Part model, mm, in its own coordinate system. Face numbers are marked on the shaded views. A direction names the side the tool comes from. Round coordinates to 2 decimals unless told otherwise and drop trailing zeros. Order: outer loops, then holes, each group sorted by start corner. A loop starts at its lowest first (then second) coordinate and runs counter-clockwise, first axis right, second up. Notation, with made-up numbers: (14, 21) -> (29, 21) arc R5 cw to (29, 30) -> close; hole circle Ø11 at (75, 31). An arc over 180 degrees is marked (long way). Use CSV: the item, a comma, the result in double quotes.
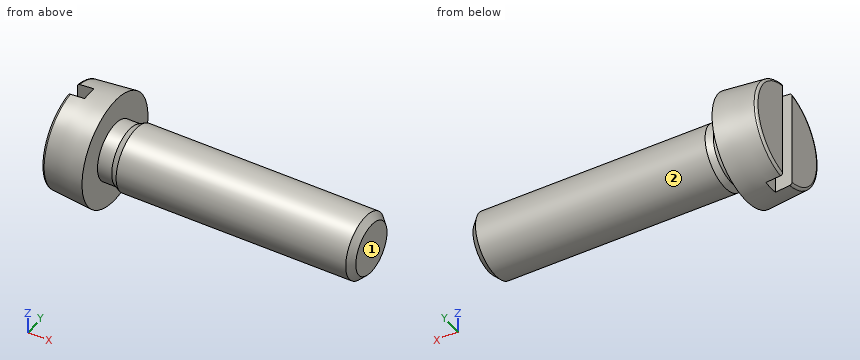
Autodesk Inventor part; units mm, degrees
ref_plane "Work Plane1" through (30.1625, 0, 0) normal (0, 0, -1) x (1, 0, 0)
ref_plane "YZ Plane" through (0, 0, 0) normal (1, 0, 0) x (0, 1, 0)
ref_plane "XZ Plane" through (0, 0, 0) normal (0, 1, 0) x (-1, 0, 0)
sketch "Sketch1" plane through (0, 0, 0) normal (0, 0, 1) x (1, 0, 0)
  line L0 (-3.3, 0) -> (20, 0)
  line L1 (20, 0) -> (20, 2.5)
  line L2 (20, 2.5) -> (1.6, 2.5)
  line L3 (1.6, 2.5) -> (1.1091, 2.2547)
  line L4 (1.1091, 2.2547) -> (0, 2.2547)
  line L5 (0, 2.2547) -> (0, 4.25)
  line L6 (-7.96, 0) -> (24.66, 0)
  line L7 (0, -0.85) -> (0, 5.1)
  line L8 (-3.3, 0) -> (-3.3, 3.9613)
  line L9 (0, 4.25) -> (-3.3, 3.9613)
  line L10 (1.6, 2.5) -> (0, 2.5) construction
  dimension "d0" = 20
  dimension "d1" = 18.4
  dimension "d2" = 0.4909
  dimension "d3" = 3.3
  dimension "d4" = 5
  dimension "d5" = 4.5095
  dimension "d9" = 8.5
  dimension "d10" = 5
revolve "Body" add sketch "Sketch1" angle 360 about axis through (-3.3, 0, 0) along (1, 0, 0)
sketch "Sketch2" plane through (-3.3, 0, 0) normal (-1, 0, 0) x (0, 0, 1)
  circle A0 centre (0, 0) radius 4.25
  line L0 (0, 0) -> (0, 3.9613)
  line L1 (-4.25, 0.6) -> (4.25, 0.6)
  line L2 (4.25, 0.6) -> (4.25, -0.6)
  line L3 (4.25, -0.6) -> (-4.25, -0.6)
  line L4 (-4.25, -0.6) -> (-4.25, 0.6)
  line L5 (-4.25, 0) -> (4.25, 0) construction
  line L6 (0, 0.6) -> (0, -0.6) construction
  point P0 (0, 0)
  dimension "d11" = 1.2
  dimension "d12" = 8.5
fillet "Fillet1" radius 0.2 1 edges at (-3.3, -3.9613, 0)
extrude "Slot" cut sketch "Sketch2" against normal blind 1.3 contours A0 L3 L1 | L2 L3 A0 | A0 L1 L2 | A0 L4 L1 | L3 L4 A0
thread "Thread"
chamfer "Chamfer1" distance 0.4908 distance2 0.4909 1 edges at (20, -2.5, 0) measured on face at (20, 1.2612, -0.6619)
ref_plane "Work Plane1" through (30.1625, 0, 0) normal (0, 0, -1) x (1, 0, 0)
equation "\"d11\" = SBR"
equation "\"d12\" = KOD"
equation "\"d19\" = STI"
equation "\"d14\" = RR"
equation "\"d15\" = GEL"
equation "\"d17\" = -0.5 * SPD + 0.5 * GD"
equation "\"d0\" = NLG"
equation "\"d1\" = GEL"
equation "\"d3\" = KOH"
equation "\"d4\" = GD"
equation "\"d5\" = BDM"
equation "\"d9\" = KOD"
equation "\"d10\" = KEWI"
equation "\"GD\" = NND"
equation "\"NLG\" = 20"
equation "\"GEL\" = 18.4"
equation "\"KOD\" = 8.5"
equation "\"KOH\" = 3.3"
equation "\"GAL\" = 0.61345 * PTC"
equation "\"SPD\" = NND - 1.2269 * PTC"
equation "\"BDM\" = 4.5095"
equation "\"GUL\" = 0.61345 * PTC"
equation "\"RR\" = 0.2"
equation "\"SBR\" = 1.2"
equation "\"STI\" = 1.3"
equation "\"KEWI\" = 5deg"
equation "\"PTC\" = 0.8"
equation "\"THREADDIA\" = 5"
equation "\"TOA\" = 30deg"
equation "\"NND\" = 5"
equation "\"GD1\" = THREADDIA - 1.2269 * PTC"
properties part number "ISO 1207 - M5 x 20" material "Stainless Steel, 440C"
(1) Cut at B-B, the plane z = 0. Give the cut face in (x, y), then the cut area to 3 significant figures.
Reply:
outline,"(-3.3, -3.78) arc R0.2 ccw to (-3.12, -3.98) -> (0, -4.25) -> (0, -2.25) -> (1.11, -2.25) -> (1.6, -2.5) -> (19.51, -2.5) -> (20, -2.01) -> (20, 2.01) -> (19.51, 2.5) -> (1.6, 2.5) -> (1.11, 2.25) -> (0, 2.25) -> (0, 4.25) -> (-3.12, 3.98) arc R0.2 ccw to (-3.3, 3.78) -> (-3.3, 0.6) -> (-2, 0.6) -> (-2, -0.6) -> (-3.3, -0.6) -> close"
area,"125 mm2"
(2) Cut at C-C, the plane x = -1.25. Give the cut face in (y, z).
Reply:
outline,"circle Ø8.28 at (0, 0)"
(3) Probe probe 1 along X at (y, z) = (-1, 2.5); probe 2 along X at (y, z) = (1, 2.25); probe 3 along Y at (x, z) = (8, 2.25). List the from-to ranges inside material, lowest first. Write a range as [from, to].
Reply:
probe 1,"[-3.3, 0]"
probe 2,"[-3.3, 0], [1.52, 19.55]"
probe 3,"[-1.09, 1.09]"
(4) Cut at A-A, the plane y = 0. Give the cut face in (x, z).
Reply:
outline,"(-2, -4.08) -> (0, -4.25) -> (0, -2.25) -> (1.11, -2.25) -> (1.6, -2.5) -> (19.51, -2.5) -> (20, -2.01) -> (20, 2.01) -> (19.51, 2.5) -> (1.6, 2.5) -> (1.11, 2.25) -> (0, 2.25) -> (0, 4.25) -> (-2, 4.08) -> close"
(5) Which spindle directions (+Z, -Z, +X, -X, +Y, -Y) get a long thin tool onto all of the face, cutting with end or side? Do the marked faces 1 and 2. Say none if no direction does.
Reply:
face 1,"+Z, -Z, +X, +Y, -Y"
face 2,"+X"
(6) Drop flat-ended pins along their axis: P1, Ø1.4, axis at x = -2.5, z = 1.5, coming from the -Y side; P2, Ø2, axis at y = -3, z = 0.5, coming from the +X side; P3, Ø1, axis at y = 0, z = -2, coming from the -X side. Give the stop position or say it passes through.
Reply:
P1,"y = -3.96"
P2,"x = 19.97"
P3,"x = -2"
